The listing builds one solid part. Answer for the finished solid, in the listing's coordinates (mm). A direction names the side the tool comes from. Round coordinates to 2 decimals unless told otherwise and drop trailing zeros. Loops run counter-clockwise (first coordinate to the right, second up) from the corner with the lowest first, then second, coordinate; pieces in that order, holes last. Notation, with made-up numbers: (-30.5, -37.75) -> (6.5, -37.75) arc R22 cw to (6.5, -26.75) -> close; hole circle Ø9 at (41.25, -11). An arc over 180 degrees is marked (long way). Use a Markdown table: item, result. Add a question column.
Q1. For a pull along X with two mould halves and no side action, classify faces 1 (the flat face through (32, -8, 19.225)), 2 (the flat face through (36.98, -5.87, 17.94)), 3 (the cylindrical face through (1.16, -5.42, 17.8)), 4 (the flat face through (35, -1.8, 17)) as released by +X, released by -X, zero draft, split by the parting line, or undercut.
Q2. Given pin 1 Ø3 at (x, z) = (14.5, 18) entering from +Y; pin 2 Ø2.5 at (x, y) = (56, -3) entering from +Z; pin 3 Ø4 at (x, y) = (27, -1) entering from +Z, each flat-ended and moving along its own axis, determine where each tip first touches the part or whether it passes through.
Q3. Consider line 1 (X direction, y = -3.5, z = 18.55); line 2 (X direction, y = -5, z = 17.8); line 3 (Z direction, x = 8.5, y = -4.75). Determine where each line is inside the solid, lowest interval first.
Q4. Section B-B on y = -8.5 is taken. Give the vertices of the cut face in (x, z), then the cut area to 3 significant figures.
Q5. Which of the six approach directions +Z, -Z, +X, -X, +Y, -Y give full straight-line access (tool end or side, diameter ignored) to faces 5 (the cylindrical face through (31.699, -1.426, 17.722)), 6 (the flat face through (57.003, -3.169, 17.645))?
Q6. Section C-C on y = -1.25 is taken. Give the vertices of the cut face in (x, z).
from build123d import *

# Parameters (mm, degrees)
F0_W        = 65
F0_H        = 5.4
F1_DEPTH    = 11
F2_W        = 65
F2_H        = 1.4
F3_DEPTH    = 1
F4_R        = 1.65
F5_DEPTH    = 25
F7_DEPTH    = 2.6
F8_T1_DEPTH = 36
F8_T3_DEPTH = 90
F9_SIZE     = 0.99999


# Not quite as in the source:
# - a fillet or chamfer that OpenCascade refuses, or shapes differently, is made with other operations: its cross-section is extruded or revolved along the edge and cut away or added
# - a fillet or chamfer is up to 0.001 mm smaller than in the source, because OpenCascade refuses the exact size


with BuildPart() as f1:
    # F0 (on Front) → F1 (new body)
    with BuildSketch(Plane.XZ):
        with Locations((32.1536201239, 16.5253020123)):
            Rectangle(F0_W, F0_H)
    extrude(amount=F1_DEPTH)

    # F2 (on face) → F3 (cut)
    with BuildSketch(Plane.XZ.offset(11)):
        with Locations((32.1536201239, 16.5253020123)):
            Rectangle(F2_W, F2_H)
    extrude(amount=-F3_DEPTH, mode=Mode.SUBTRACT)

    # F4 (on face) → F5 (cut)
    with BuildSketch(Plane.XY.offset(19.2253020123)):
        with Locations((14.6536201239, -4.5)):
            Circle(F4_R)
        with Locations((34.6536201239, -4.5)):
            Circle(F4_R)
        with Locations((54.6536201239, -4.5)):
            Circle(F4_R)
    extrude(amount=-F5_DEPTH, mode=Mode.SUBTRACT)

    # F6 (on face) → F7 (cut)
    with BuildSketch(Plane.XY.offset(19.2253020123)):
        Polygon((13.0947743971, -7.2), (16.2124658507, -7.2), (17.7713115775, -4.5), (16.2124658507, -1.8), (13.0947743971, -1.8), (11.5359286702, -4.5), align=None)
        Polygon((33.0947743971, -7.2), (36.2124658507, -7.2), (37.7713115775, -4.5), (36.2124658507, -1.8), (33.0947743971, -1.8), (31.5359286702, -4.5), align=None)
        Polygon((53.0947743971, -7.2), (56.2124658507, -7.2), (57.7713115775, -4.5), (56.2124658507, -1.8), (53.0947743971, -1.8), (51.5359286702, -4.5), align=None)
    extrude(amount=-F7_DEPTH, mode=Mode.SUBTRACT)

    # F8: fillet of radius 5 on 3 edges, made by hand

    # F8_s2 → F8_t1 (cut)
    with BuildSketch(Plane.XZ.offset(-12.5)):
        with BuildLine():
            ThreePointArc((64.6536201239, 14.2253020123), (63.1891540298, 17.7608359182), (59.6536201239, 19.2253020123))
            Line((59.6536201239, 19.2253020123), (64.6536201239, 19.2253020123))
            Line((64.6536201239, 19.2253020123), (64.6536201239, 14.2253020123))
        make_face()
        with BuildLine():
            ThreePointArc((4.6536201239, 19.2253020123), (1.1180862179, 17.7608359182), (-0.3463798761, 14.2253020123))
            Line((-0.3463798761, 14.2253020123), (-0.3463798761, 19.2253020123))
            Line((-0.3463798761, 19.2253020123), (4.6536201239, 19.2253020123))
        make_face()
    extrude(amount=F8_T1_DEPTH, mode=Mode.SUBTRACT)

    # F8_s4 → F8_t3 (cut)
    with BuildSketch(Plane.YZ.offset(-12.8463798761)):
        with BuildLine():
            ThreePointArc((0, 14.2253020123), (-1.4644660941, 17.7608359182), (-5, 19.2253020123))
            Line((-5, 19.2253020123), (0, 19.2253020123))
            Line((0, 19.2253020123), (0, 14.2253020123))
        make_face()
    extrude(amount=F8_T3_DEPTH, mode=Mode.SUBTRACT)

    # F9 (size 1 in the source; OpenCascade refuses exactly that, so slightly less here)
    f9_edges = [f1.edges().sort_by_distance(p)[0] for p in [
        (32.15362, -11, 17.225302),
    ]]
    chamfer(f9_edges, length=F9_SIZE)


solid = f1.part
Checked values:
| question | item | result |
|---|---|---|
| 1 | face 1 | zero draft |
| 1 | face 2 | undercut |
| 1 | face 3 | released by -X |
| 1 | face 4 | undercut |
| 2 | pin 1 | stops at y = -0.55 |
| 2 | pin 2 | stops at z = 18.98 |
| 2 | pin 3 | stops at z = 18.81 |
| 3 | line 1 | x = 2.14 to 12.11, 17.19 to 32.11, 37.19 to 52.11, 57.19 to 62.16 |
| 3 | line 2 | x = 1.16 to 11.82, 17.48 to 31.82, 37.48 to 51.82, 57.48 to 63.15 |
| 3 | line 3 | z = 13.83 to 19.22 |
| 4 | outline | (-0.35, 13.83) -> (64.65, 13.83) -> (64.65, 14.23) arc R5 ccw to (59.65, 19.23) -> (4.65, 19.23) arc R5 ccw to (-0.35, 14.23) -> close |
| 4 | area | 340 mm2 |
| 5 | face 5 | +Z, +X, -X, +Y |
| 5 | face 6 | +Z |
| 6 | outline | (-0.35, 13.83) -> (64.65, 13.83) -> (64.65, 14.23) arc R5 ccw to (63.4, 17.53) -> (0.9, 17.53) arc R5 ccw to (-0.35, 14.23) -> close |
